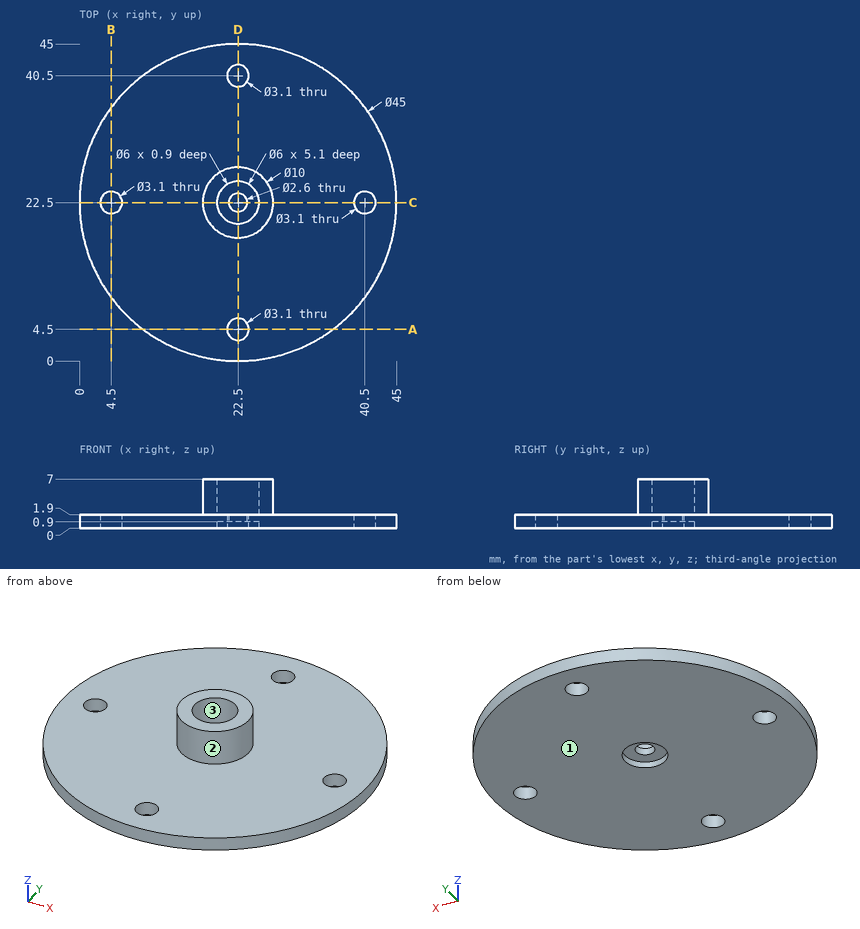
Answer from the drawing. Dimensions are ordinates in mm from the lowest x, y and z of the part. Coordinates: 2 decimals unless noted, no trailing zeros. Loops run counter-clockwise (first coordinate to the right, second up) from the corner with the lowest first, then second, coordinate; pieces in that order, holes last.
Q1. The part is cut by section A-A on y = 4.5. Write down the section's boundary in (x, z), and give its area (3 significant figures).
Q2. Consider probe 1 along Y at (x, z) = (22.5, 1.4); probe 2 along Y at (x, z) = (22.5, 0.45); probe 3 along Z at (x, y) = (7.5, 32.5). Determine where each line is inside the solid, lowest interval first.
Q3. The part is cut by section C-C on y = 22.5. Write down the section's boundary in (x, z), and give its area (3 significant figures).
Q4. Each of these flat-tipped pins is pushed along its axis until it touches: pin 1 Ø5 at (x, y) = (24, 23) entering from +Z; pin 2 Ø1.5 at (x, z) = (9, 2.5) entering from +Y; pin 3 Ø3 at (x, y) = (4.5, 22.5) entering from +Z; pin 4 Ø1 at (x, y) = (34.5, 8) entering from +Z. Where does it stop, or does it pass through?
Q5. The mould has two halves that part along X. Classify the marked faces 1, 2 and 3: +X half, -X half, draft (parallel to the pull), parting line (faces both ways), or undercut.
Results below:
1. outline: (9, 0) - (20.95, 0) - (20.95, 1.9) - (9, 1.9) - close; (24.05, 0) - (36, 0) - (36, 1.9) - (24.05, 1.9) - close
1. area: 45.4 mm2
2. probe 1: y = 0 to 2.95, 6.05 to 21.2, 23.8 to 38.95, 42.05 to 45
2. probe 2: y = 0 to 2.95, 6.05 to 19.5, 25.5 to 38.95, 42.05 to 45
2. probe 3: z = 0 to 1.9
3. outline: (0, 0) - (2.95, 0) - (2.95, 1.9) - (0, 1.9) - close; (6.05, 0) - (19.5, 0) - (19.5, 0.9) - (21.2, 0.9) - (21.2, 1.9) - (19.5, 1.9) - (19.5, 7) - (17.5, 7) - (17.5, 1.9) - (6.05, 1.9) - close; (23.8, 0.9) - (25.5, 0.9) - (25.5, 0) - (38.95, 0) - (38.95, 1.9) - (27.5, 1.9) - (27.5, 7) - (25.5, 7) - (25.5, 1.9) - (23.8, 1.9) - close; (42.05, 0) - (45, 0) - (45, 1.9) - (42.05, 1.9) - close
3. area: 86.1 mm2
4. pin 1: stops at z = 7
4. pin 2: stops at y = 40.83
4. pin 3: passes through
4. pin 4: stops at z = 1.9
5. face 1: draft
5. face 2: parting line
5. face 3: undercut
